For this review, take the finished solid that the model builds, in its own axes (mm). A direction names the side the tool comes from. Round coordinates to 2 decimals unless told otherwise and drop trailing zeros. Order: outer loops, then holes, each group sorted by start corner. A loop starts at its lowest first (then second) coordinate and runs counter-clockwise, first axis right, second up. Notation, with made-up numbers: (59, 76) - (90, 76) arc R38 ccw to (90, 114) - close; hole circle Ø4 at (46.25, 44.25). An arc over 180 degrees is marked (long way). Write each question's results on one line, items separated by ' | '. Start each with the question number.
(1) Draft analysis for pull direction Y (two halves, no side actions). For faces 6 (the cylindrical face through (171.93, 16.37, -4.93)), 7 (the flat face through (76, 37.5, -67)), 8 (the cylindrical face through (106.034, 41.972, -20.479)), 9 (the flat face through (30, 44, -23)), state which applies: pulls with the +Y half, pulls with the -Y half, needs draft (parallel to the pull), parting line crosses it, or undercut.
(2) For faces 1 (the flat face through (76, 44, -23)), 2 (the flat face through (76, 37.5, -19)), 3 (the flat face through (10, 27, -85)), 4 (the cylindrical face through (12.05, 16.2, 2.77)), 5 (the cylindrical face through (108.799, 41.972, -68.815)), list the 3-axis set-ups (+Z, -Z, +X, -X, +Y, -Y) from which the entire face can be reached by the end or side of a thin tool; tool diameter is ignored.
(3) For L1, parallel to Y at x = 15, z = -4.5; L2, parallel to X at y = 39, z = -21; L3, parallel to X at y = 42.5, z = -61.5, list the stretches that pass through material, from the lowest coordinate up. Write a range as from..to.
(4) Take a section at A-A, the plane y = 13.5. Give the boundary of the cut face in (x, z), plus the area to 3 significant figures.
(5) Insertion check: pin 1 Ø1.5 at (x, y) = (64, 32.5) entering from -Z; pin 2 Ø6 at (x, z) = (156, -22) entering from -Y; pin 3 Ø2 at (y, z) = (13.5, -9.5) entering from -X; pin 4 Ø2 at (x, z) = (110, -21) entering from -Y. Each pin has a flat end and moves straight along its axis. Give the tip position at first contact, or say it passes through.
(6) Take a section at C-C, the plane z = -52. Give the boundary of the cut face in (x, y).
(7) Take a section at B-B, the plane x = 190. Give the boundary of the cut face in (y, z).
(8) Take a section at D-D, the plane x = 137. Give the boundary of the cut face in (y, z), plus the area to 3 significant figures.
```python
from build123d import *

# Parameters (mm, degrees)
BODY_DEPTH                        = 200
SKETCH4_R                         = 7.5
MOUNTING_NOBS_DEPTH               = 10
SIDE_MOUNTING_HOLES_START         = -10
SIDE_MOUNTING_HOLES_OUTLINE_R     = 2.25
SIDE_MOUNTING_HOLES_DEPTH         = 15
SIDE_MOUNTING_HOLES_START_2       = 0.6
SIDE_MOUNTING_HOLES_2_OUTLINE_R   = 4
SIDE_MOUNTING_HOLES_2_OUTLINE_R_2 = 2.25
SIDE_MOUNTING_HOLES_2_DEPTH       = 4.4
SKETCH8_R                         = 4
DC_DRIVER_NOBS_DEPTH              = 4
DC_DRIVER_MOUNTING_START          = 35
DC_DRIVER_MOUNTING_OUTLINE_R      = 1.7
DC_DRIVER_MOUNTING_DEPTH          = 9
DC_DRIVER_NUT_CUTS_DEPTH          = 2.5
DC_DRIVER_PATTERN_COUNT           = 2
DC_DRIVER_PATTERN_PITCH           = 80
SKETCH13_R                        = 5
SUPPORT_NOBS_DEPTH                = 8


# Read off the part's stored shape, not the designer's step: side_mounting_holes, dc_driver_mounting
with BuildPart() as part:
    # Sketch1 → body (new body)
    with BuildSketch(Plane(origin=(0, 0, 0), x_dir=(0, 0, -1), z_dir=(1, 0, 0))):
        Polygon((0, 0), (0, 35), (95, 35), (95, 40), (-5, 40), (-5, 0), align=None)
    extrude(amount=BODY_DEPTH)

    # Sketch4 → mounting_nobs (add)
    with BuildSketch(Plane(origin=(0, 0, 0), x_dir=(-1, 0, 0), z_dir=(0, 0, -1))):
        with Locations(Location((-165, 13.5, 0), (0, 0, 180))):
            Circle(SKETCH4_R)
        with Locations(Location((-15, 13.5, 0), (0, 0, 180))):
            Circle(SKETCH4_R)
    extrude(amount=MOUNTING_NOBS_DEPTH)

    # side_mounting_holes outline → side_mounting_holes (cut)
    with BuildSketch(Plane.XY.offset(SIDE_MOUNTING_HOLES_START)):
        with Locations((165, 13.5)):
            Circle(SIDE_MOUNTING_HOLES_OUTLINE_R)
        with Locations((15, 13.5)):
            Circle(SIDE_MOUNTING_HOLES_OUTLINE_R)
    extrude(amount=SIDE_MOUNTING_HOLES_DEPTH, mode=Mode.SUBTRACT)

    # side_mounting_holes 2 outline → side_mounting_holes 2 (cut)
    # profile 1 of 2: a face of its own
    with BuildSketch(Plane.XY.offset(SIDE_MOUNTING_HOLES_START_2)):
        with Locations((165, 13.5)):
            Circle(SIDE_MOUNTING_HOLES_2_OUTLINE_R)
        with Locations((165, 13.5)):
            Circle(SIDE_MOUNTING_HOLES_2_OUTLINE_R_2, mode=Mode.SUBTRACT)
    # profile 2 of 2: a face of its own
    with BuildSketch(Plane.XY.offset(SIDE_MOUNTING_HOLES_START_2)):
        with Locations((15, 13.5)):
            Circle(SIDE_MOUNTING_HOLES_2_OUTLINE_R)
        with Locations((15, 13.5)):
            Circle(SIDE_MOUNTING_HOLES_2_OUTLINE_R_2, mode=Mode.SUBTRACT)
    extrude(amount=SIDE_MOUNTING_HOLES_2_DEPTH, mode=Mode.SUBTRACT)

    # Sketch8 → dc_driver_nobs (add)
    with BuildSketch(Plane(origin=(0, 40, 0), x_dir=(1, 0, 0), z_dir=(0, 1, 0))):
        with Locations(Location((30, 65, 0), (0, 0, 90))):
            Circle(SKETCH8_R)
        with Locations(Location((75.9, 65, 0), (0, 0, 90))):
            Circle(SKETCH8_R)
        with Locations(Location((30, 21, 0), (0, 0, 90))):
            Circle(SKETCH8_R)
        with Locations(Location((75.9, 21, 0), (0, 0, 90))):
            Circle(SKETCH8_R)
    dc_driver_nobs = extrude(amount=DC_DRIVER_NOBS_DEPTH)

    # dc_driver_mounting outline → dc_driver_mounting (cut)
    with BuildSketch(Plane(origin=(0, 0, 0), x_dir=(1, 0, 0), z_dir=(0, 1, 0)).offset(DC_DRIVER_MOUNTING_START)):
        with Locations((75.9, 65)):
            Circle(DC_DRIVER_MOUNTING_OUTLINE_R)
        with Locations((30, 21)):
            Circle(DC_DRIVER_MOUNTING_OUTLINE_R)
        with Locations((75.9, 21)):
            Circle(DC_DRIVER_MOUNTING_OUTLINE_R)
        with Locations((30, 65)):
            Circle(DC_DRIVER_MOUNTING_OUTLINE_R)
    dc_driver_mounting = extrude(amount=DC_DRIVER_MOUNTING_DEPTH, mode=Mode.SUBTRACT)

    # Sketch12 → dc_driver_nut_cuts (cut)
    with BuildSketch(Plane.XZ.offset(-35)):
        Polygon((33.117691454, -21), (31.558845727, -18.3), (28.441154273, -18.3), (26.882308546, -21), (28.441154273, -23.7), (31.558845727, -23.7), align=None)
        Polygon((79.017691454, -21), (77.458845727, -18.3), (74.341154273, -18.3), (72.782308546, -21), (74.341154273, -23.7), (77.458845727, -23.7), align=None)
        Polygon((79.017691454, -65), (77.458845727, -62.3), (74.341154273, -62.3), (72.782308546, -65), (74.341154273, -67.7), (77.458845727, -67.7), align=None)
        Polygon((33.117691454, -65), (31.558845727, -62.3), (28.441154273, -62.3), (26.882308546, -65), (28.441154273, -67.7), (31.558845727, -67.7), align=None)
    dc_driver_nut_cuts = extrude(amount=-DC_DRIVER_NUT_CUTS_DEPTH, mode=Mode.SUBTRACT)

    # dc_driver_pattern: dc_driver_nobs, dc_driver_mounting, dc_driver_nut_cuts ×2
    with Locations(*[(i * DC_DRIVER_PATTERN_PITCH, 0, 0) for i in range(1, DC_DRIVER_PATTERN_COUNT)]):
        add(dc_driver_nobs)
        add(dc_driver_mounting, mode=Mode.SUBTRACT)
        add(dc_driver_nut_cuts, mode=Mode.SUBTRACT)

    # Sketch13 → support_nobs (add)
    with BuildSketch(Plane.XZ.offset(-35)):
        with Locations(Location((10, -85, 0), (0, 0, 90))):
            Circle(SKETCH13_R)
        with Locations(Location((190, -85, 0), (0, 0, 90))):
            Circle(SKETCH13_R)
    extrude(amount=SUPPORT_NOBS_DEPTH)


solid = part.part
```
Results below:
1) face 6: undercut | face 7: pulls with the -Y half | face 8: needs draft | face 9: pulls with the +Y half
2) face 1: +Z, -Z, +X, -X, +Y | face 2: -Y | face 3: -Z, +X, -X, -Y | face 4: +Z | face 5: +Y
3) L1: y = 6..11.25, 15.75..21, 35..40 | L2: x = 0..28.3, 31.7..74.2, 77.6..108.3, 111.7..154.2, 157.6..200 | L3: x = 28.06..31.94, 73.96..77.84, 108.06..111.94, 153.96..157.84
4) outline: (0, 0) - (7.5, 0) - (7.5, -10) - (12.75, -10) - (12.75, 0.6) - (11, 0.6) - (11, 5) - (0, 5) - close; (17.25, -10) - (22.5, -10) - (22.5, 0) - (157.5, 0) - (157.5, -10) - (162.75, -10) - (162.75, 0.6) - (161, 0.6) - (161, 5) - (19, 5) - (19, 0.6) - (17.25, 0.6) - close; (167.25, -10) - (172.5, -10) - (172.5, 0) - (200, 0) - (200, 5) - (169, 5) - (169, 0.6) - (167.25, 0.6) - close | area: 1,130 mm^2
5) pin 1: stops at z = 0 | pin 2: stops at y = 35 | pin 3: stops at x = 7.5 | pin 4: passes through
6) outline: (0, 35) - (200, 35) - (200, 40) - (0, 40) - close
7) outline: (0, 0) - (35, 0) - (35, -80) - (27, -80) - (27, -90) - (35, -90) - (35, -95) - (40, -95) - (40, 5) - (0, 5) - close
8) outline: (0, 0) - (35, 0) - (35, -95) - (40, -95) - (40, 5) - (0, 5) - close | area: 675 mm^2
